Geometry: final body of the model. Coordinates: model frame, mm. A direction names the side the tool comes from. Give positions to 0.01 mm unless a question says otherwise; leave off trailing zeros. Write each loop counter-clockwise with the first axis right and the second up, starting at its lowest first coordinate (ties: lowest second). Pieces come first, ordered by that corner, then holes.
from build123d import *

# Parameters (mm, degrees)
SKETCH_1_W             = 12.6
SKETCH_1_H             = 18.4
EXTRUDE_1_DEPTH        = 11
SKETCH_2_W             = 15
SKETCH_2_H             = 21
EXTRUDE_2_DEPTH        = 2
FILLET_1_R             = 0.5
EXTRUDE_3_DEPTH        = 5
SKETCH_4_W             = 5
SKETCH_4_H             = 0.6
EXTRUDE_4_DEPTH        = 8
PATTERN_LINEAR_1_COUNT = 2
PATTERN_LINEAR_1_PITCH = 6.8


with BuildPart() as part:
    # Эскиз1 → Бобышка-Вытянуть1 (new body)
    with BuildSketch(Plane.XY):
        Rectangle(SKETCH_1_W, SKETCH_1_H)
    extrude(amount=EXTRUDE_1_DEPTH)

    # Эскиз2 → Бобышка-Вытянуть2 (add)
    with BuildSketch(Plane.XY.offset(11)):
        Rectangle(SKETCH_2_W, SKETCH_2_H)
    extrude(amount=EXTRUDE_2_DEPTH)

    # Скругление1
    fillet_1_edges = [part.edges().sort_by_distance(p)[0] for p in [
        (7.5, 0, 13),
        (0, 10.5, 13),
        (-7.5, 0, 13),
        (0, -10.5, 13),
    ]]
    fillet(fillet_1_edges, radius=FILLET_1_R)

    # Эскиз3 → Бобышка-Вытянуть3 (add, symmetric)
    with BuildSketch(Plane(origin=(0, 0, 0), x_dir=(0, 0, -1), z_dir=(1, 0, 0))):
        with BuildLine():
            Line((-13, -7.7), (-13, 7.7))
            ThreePointArc((-13, 7.7), (-15.160810119, 7.050490206), (-16.8, 5.5))
            ThreePointArc((-16.8, 5.5), (-13.968906968, -0.831958067), (-13, -7.7))
        make_face()
    extrude(amount=EXTRUDE_3_DEPTH, both=True)

    # Эскиз4 → Бобышка-Вытянуть4 (add)
    with BuildSketch(Plane(origin=(0, 0, 0), x_dir=(-1, 0, 0), z_dir=(0, 0, -1))):
        Rectangle(SKETCH_4_W, SKETCH_4_H)
    extrude_4 = extrude(amount=EXTRUDE_4_DEPTH)

    # Линейный массив1: Бобышка-Вытянуть4 ×2
    with Locations(*[(0, i * PATTERN_LINEAR_1_PITCH, 0) for i in range(1, PATTERN_LINEAR_1_COUNT)]):
        add(extrude_4)


solid = part.part
Q1. Ray query, line 1 along Y through (x, z) = (-2, -5); line 2 along X through (y, z) = (5.25, 4.5); line 3 along X through (y, z) = (6.25, 15.5). Return the intervals inside material, ascending.
Filled sheet:
line 1: y = -0.3 to 0.3, 6.5 to 7.1
line 2: x = -6.3 to 6.3
line 3: x = -5 to 5
Q2. Section D-D on x = -6. Output: boundary loops of the cut face in (y, z).
Filled sheet:
outline: (-10.5, 11) - (-9.2, 11) - (-9.2, 0) - (9.2, 0) - (9.2, 11) - (10.5, 11) - (10.5, 12.5) arc R0.5 ccw to (10, 13) - (-10, 13) arc R0.5 ccw to (-10.5, 12.5) - close
Q3. Section A-A on z = -3. Output: boundary loops of the cut face in (x, y), plus the area to 3 significant figures.
Filled sheet:
outline: (-2.5, -0.3) - (2.5, -0.3) - (2.5, 0.3) - (-2.5, 0.3) - close; (-2.5, 6.5) - (2.5, 6.5) - (2.5, 7.1) - (-2.5, 7.1) - close
area: 6.00 mm2
Q4. Pin query (flat end, axial travel): P1, Ø6.5, axis at x = 0.5, y = -4.5, coming from the -Z side; P2, Ø5, axis at x = 4, y = -4, coming from the +Z side; P3, Ø4, axis at x = -1, z = -3, coming from the +Y side. Return the tip coordinate at first contact, or that it passes through.
Filled sheet:
P1: stops at z = 0
P2: stops at z = 13.79
P3: stops at y = 7.1
Q5. Pull-direction query (Y, two-part tool) for faces 5 (the flat face through (0, 0.3, -4)), 6 (the flat face through (7.5, 0, 12)), 7 (the flat face through (0, 6.5, -4)), 8 (the flat face through (0, -9.2, 5)); classes: released by +Y, released by -Y, zero draft, split by the parting line, or undercut.
Filled sheet:
face 5: undercut
face 6: zero draft
face 7: undercut
face 8: released by -Y
Q6. Section B-B on x = -1.5. Output: boundary loops of the cut face in (y, z).
Filled sheet:
outline: (-10.5, 11) - (-9.2, 11) - (-9.2, 0) - (-0.3, 0) - (-0.3, -8) - (0.3, -8) - (0.3, 0) - (6.5, 0) - (6.5, -8) - (7.1, -8) - (7.1, 0) - (9.2, 0) - (9.2, 11) - (10.5, 11) - (10.5, 12.5) arc R0.5 ccw to (10, 13) - (7.7, 13) arc R4.89 ccw to (5.5, 16.8) arc R24.83 cw to (-7.7, 13) - (-10, 13) arc R0.5 ccw to (-10.5, 12.5) - close
Q7. Section C-C on y = 0. Output: boundary loops of the cut face in (x, z), plus the area to 3 significant figures.
Filled sheet:
outline: (-7.5, 11) - (-6.3, 11) - (-6.3, 0) - (-2.5, 0) - (-2.5, -8) - (2.5, -8) - (2.5, 0) - (6.3, 0) - (6.3, 11) - (7.5, 11) - (7.5, 12.5) arc R0.5 ccw to (7, 13) - (5, 13) - (5, 14.22) - (-5, 14.22) - (-5, 13) - (-7, 13) arc R0.5 ccw to (-7.5, 12.5) - close
area: 221 mm2
Q8. Access query for faces 1 (the flat face through (6.3, 0, 5)), 2 (the flat face through (-6.3, 0, 5)), 3 (the flat face through (-6, 0, 13)), 4 (the flat face through (0, -0.3, -4)). Directions: +Z, -Z, +X, -X, +Y, -Y. A direction counts if a zero-diameter tool reaches every point of the face in a straight line with its end or side. Return the directions, or none.
Filled sheet:
face 1: -Z, +X, +Y, -Y
face 2: -Z, -X, +Y, -Y
face 3: +Z
face 4: -Z, +X, -X, -Y
